Check sheet for the drawn part. Datum: minimum x, y, z corner. Units: mm. Coordinates: 2 decimals unless noted, no trailing zeros. Order: outer loops, then holes, each group sorted by start corner. A loop starts at its lowest first (then second) coordinate and runs counter-clockwise, first axis right, second up. Notation, with made-up numbers: (-40, -3) - (-23, -3) arc R28 cw to (-23, 19) - close; hole circle Ø4 at (8.25, 28). An arc over 180 degrees is marked (long way). Return JSON: item names as keys, results as strings. Group by question number.
Item 1: Draft check along X on the marked faces 1, 2 and 3. Enter one of: pulls with the +X half, pulls with the -X half, needs draft (parallel to the pull), parting line crosses it, or undercut.
Item 2: Section check C-C on y = 4.5. Enter the section's corners in (x, z) (1 decimal), then the cut area to 3 significant figures.
Item 3: Scan lines: probe 1 along Y at (x, z) = (5, 13); probe 2 along Z at (x, y) = (27, 5) (1 decimal); probe 3 along Z at (x, y) = (25, 16) (1 decimal). Record each from-to range of solid material in increasing order.
Item 4: Section check B-B on x = 31.5. Enter the section's corners in (y, z) (1 decimal).
Item 5: Section check A-A on z = 23. Enter the section's corners in (x, y) (1 decimal), then the cut area to 3 significant figures.
Item 6: Section check D-D on y = 10.5. Enter the section's corners in (x, z) (1 decimal).
Item 7: Gauge pin test, flat ends, axial feed: pin 1 (10 mm diameter, centred on y = 3.5, z = 27.5, fed in from -X); pin 2 (10 mm diameter, centred on y = 8, z = 35, fed in from -X); pin 3 (2 mm diameter, centred on x = 6.5, z = 25, fed in from +Y); pin 4 (4.5 mm diameter, centred on x = 27.05, z = 27.05, fed in from -Y). Record the tip position at first contact, or that the pin passes through.
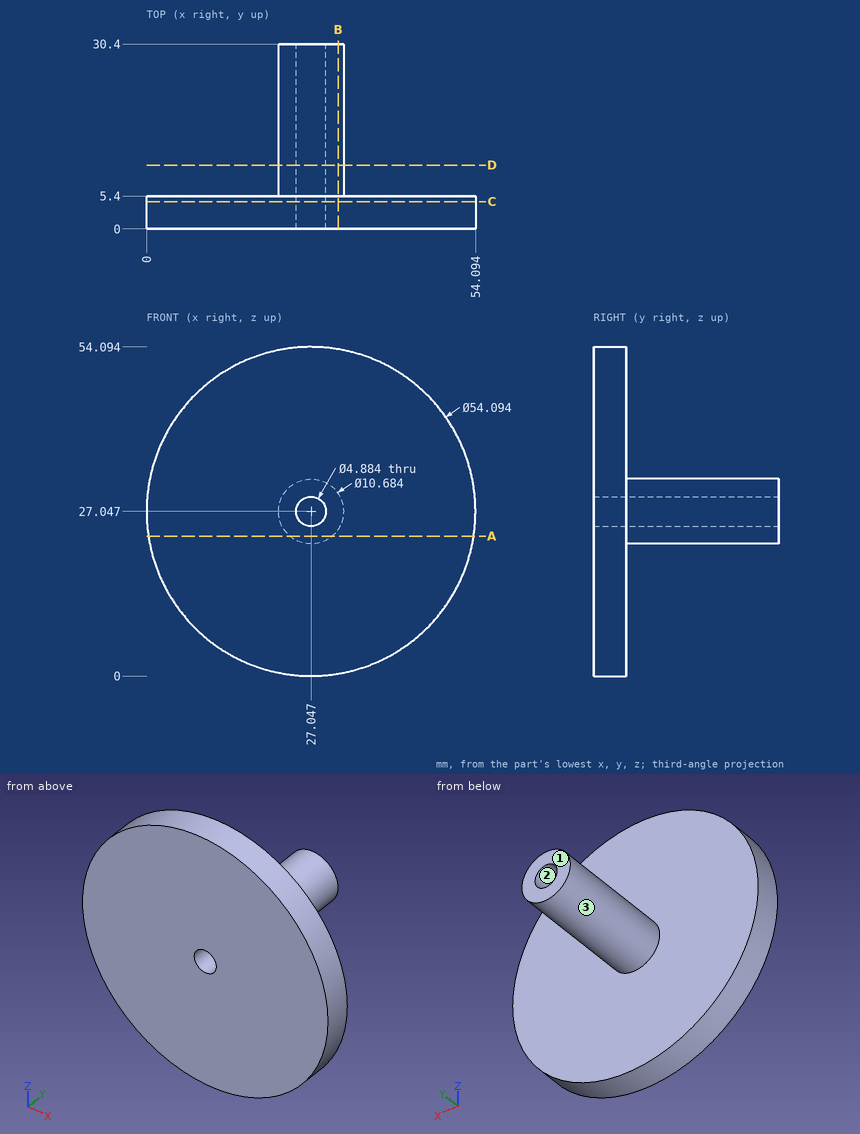
Computed:
{
 "1": {"face 1": "needs draft", "face 2": "undercut", "face 3": "parting line crosses it"},
 "2": {"outline": "circle Ø54.1 at (27, 27); hole circle Ø4.9 at (27, 27)", "area": "2,280 mm²"},
 "3": {"probe 1": "y = 0 to 5.4", "probe 2": "z = 0 to 24.6, 29.5 to 54.1", "probe 3": "z = 22.1 to 25.7, 28.4 to 32"},
 "4": {"outline": "(0, 0.4) - (5.4, 0.4) - (5.4, 24.1) - (30.4, 24.1) - (30.4, 30) - (5.4, 30) - (5.4, 53.7) - (0, 53.7) - close"},
 "5": {"outline": "(0.3, 0) - (53.8, 0) - (53.8, 5.4) - (30.5, 5.4) - (30.5, 30.4) - (23.6, 30.4) - (23.6, 5.4) - (0.3, 5.4) - close", "area": "463 mm²"},
 "6": {"outline": "circle Ø10.7 at (27, 27); hole circle Ø4.9 at (27, 27)"},
 "7": {"pin 1": "stops at x = 0", "pin 2": "stops at x = 0.25", "pin 3": "stops at y = 5.4", "pin 4": "passes through"}
}
